Autodesk Fusion 360 part; units mm, degrees
sketch "スケッチ2" plane through (0, 0, 0) normal (0, 0, 1) x (1, 0, 0)
  line L0 (15.8, 3) -> (25, -20)
  line L1 (-25, -20) -> (-15.8, 3)
  line L2 (-13.5, -20) -> (-9.5, -10)
  line L3 (-9.5, -10) -> (9.5, -10)
  line L4 (9.5, -10) -> (13.5, -20)
  line L5 (13.5, -20) -> (25, -20)
  line L6 (-13.5, -20) -> (-25, -20)
  line L7 (-15.8, 3) -> (-12.75, 3)
  line L8 (-12.75, 3) -> (-12.75, 0)
  line L9 (-12.75, 0) -> (12.75, 0)
  line L10 (12.75, 0) -> (12.75, 3)
  line L11 (12.75, 3) -> (15.8, 3)
  dimension "d1" = 19
  dimension "d2" = 9.5
  dimension "d5" = 13
  dimension "d6" = 10
  dimension "d7" = 25.5
  dimension "d8" = 3
  dimension "d9" = 11.5
  dimension "d24" = 25
  dimension "d25" = 12.75
  dimension "d26" = 20
extrude "押し出し1" add sketch "スケッチ2" along normal blind 50
sketch "スケッチ3" plane through (0, 0, 0) normal (0, 1, 0) x (1, 0, 0)
  line L0 (5, -20) -> (5, -15)
  arc A0 (5, -15) -> (-5, -15) centre (0, -15) ccw
  line L1 (-5, -15) -> (-5, -20)
  arc A1 (-5, -20) -> (5, -20) centre (0, -20) ccw
  line L2 (0, -20) -> (0, -15) construction
  dimension "d16" = 5
  dimension "d17" = 5
extrude "押し出し2" add sketch "スケッチ3" along normal blind 16
sketch "スケッチ6" plane through (0, 0, 0) normal (1, 0, 0) x (0, 1, 0)
  circle A0 centre (10, 17.5) radius 3
  line L0 (0, 0) -> (0, 50)
  dimension "d21" = 6
  dimension "d22" = 10
extrude "押し出し4" cut sketch "スケッチ6" along normal through all and the other way through all
Could you check a few things on this model? Use its own coordinates, in mm. A direction names the side the tool comes from. Round coordinates to 2 decimals unless told otherwise and drop trailing zeros. Order: outer loops, then holes, each group sorted by start corner. A loop starts at its lowest first (then second) coordinate and runs counter-clockwise, first axis right, second up.
Q1. Please list where these lines run through material, in increasing order: probe 1 along Y at (x, z) = (2.25, 17.5); probe 2 along X at (y, z) = (-14, 42); probe 3 along Y at (x, z) = (3.5, 31).
Geometry says:
probe 1: y = -10 to 7, 13 to 16
probe 2: x = -22.6 to -11.1, 11.1 to 22.6
probe 3: y = -10 to 0
Q2. Thinking about a two-plate mould opening in X: for faces 1 (the face through (-5, 4, 17)), 2 (the face through (5, 4, 18)), 3 (the face through (0, -8, 0)), 4 (the face through (5, 14, 18)), which applies, released by +X, released by -X, zero draft, split by the parting line, or undercut?
Geometry says:
face 1: undercut
face 2: undercut
face 3: zero draft
face 4: released by +X
Q3. Imagine slicing it at A-A, the plane y = -15. List the corners of the cut face in (x, z) for me.
Geometry says:
outline: (-23, 0) - (-11.5, 0) - (-11.5, 50) - (-23, 50) - close; (11.5, 0) - (23, 0) - (23, 50) - (11.5, 50) - close
Q4. Imagine slicing it at B-B, the plane z = 17.5. List the corners of the cut face in (x, y) for me, then the cut area to 3 significant figures.
Geometry says:
outline: (-25, -20) - (-13.5, -20) - (-9.5, -10) - (9.5, -10) - (13.5, -20) - (25, -20) - (15.8, 3) - (12.75, 3) - (12.75, 0) - (5, 0) - (5, 7) - (-5, 7) - (-5, 0) - (-12.75, 0) - (-12.75, 3) - (-15.8, 3) - close; (-5, 13) - (5, 13) - (5, 16) - (-5, 16) - close
area: 732 mm2
Q5. I'm going to push flat-ended pins straight in: P1, Ø6, axis at y = -10, z = 26, coming from the +X side; P2, Ø1.5, axis at x = 13.5, z = 18, coming from the +Y side; P3, Ø4, axis at y = 4.5, z = 17.5, coming from the +X side. Where does each tip first touch, or does it pass through?
Geometry says:
P1: stops at x = 22.2
P2: stops at y = 3
P3: stops at x = 16
Q6. Imagine slicing it at C-C, the plane x = 4. List the corners of the cut face in (y, z) for me.
Geometry says:
outline: (-10, 0) - (0, 0) - (0, 12) - (16, 12) - (16, 23) - (0, 23) - (0, 50) - (-10, 50) - close; hole circle Ø6 at (10, 17.5)
Q7. Which directions (+Z, -Z, +X, -X, +Y, -Y) give clear straight access to the entire face, cutting with the end or side of a thin tool? Please do faces 5 (the face through (12.75, 1, 25)), 6 (the face through (-11.53, -15.07, 24.65)), 7 (the face through (-5, 14, 17)).
Geometry says:
face 5: +Z, -Z, +Y
face 6: +Z, -Z, -Y
face 7: +Z, -Z, -X, +Y
Q8. Imagine slicing it at D-D, the plane z = 31. List the corners of the cut face in (x, y) for me.
Geometry says:
outline: (-25, -20) - (-13.5, -20) - (-9.5, -10) - (9.5, -10) - (13.5, -20) - (25, -20) - (15.8, 3) - (12.75, 3) - (12.75, 0) - (-12.75, 0) - (-12.75, 3) - (-15.8, 3) - close
